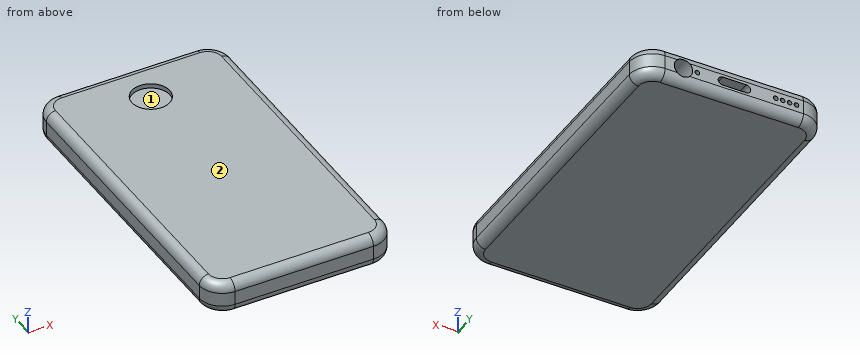
```python
from build123d import *

# Parameters (mm, degrees)
F0_W         = 40
F0_H         = 70
F1_DEPTH     = 7
F2_R         = 5
F3_R         = 2
F4_DEPTH     = 5
F5_T1_DEPTH  = 30
F5_T3_DEPTH  = 60
F5_T6_ANGLE  = 90
F5_T8_ANGLE  = 90
F5_T10_ANGLE = 90
F5_T12_ANGLE = 90
F5_T14_ANGLE = 90
F5_T16_ANGLE = 90
F5_T18_ANGLE = 90
F5_T20_ANGLE = 90
F6_R         = 4.1045895756
F7_DEPTH     = 1
F8_R         = 0.5
F9_DEPTH     = 5
F11_DEPTH    = 5
F12_R        = 0.5
F13_DEPTH    = 5


# Not quite as in the source:
# - a fillet or chamfer that OpenCascade refuses, or shapes differently, is made with other operations: its cross-section is extruded or revolved along the edge and cut away or added


with BuildPart() as f1:
    # F0 (on Top) → F1 (new body)
    with BuildSketch(Plane.XY):
        with Locations((20, 35)):
            Rectangle(F0_W, F0_H)
    extrude(amount=F1_DEPTH)

    # F2
    f2_edges = [f1.edges().sort_by_distance(p)[0] for p in [
        (40, 0, 3.5),
        (0, 0, 3.5),
        (40, 70, 3.5),
        (0, 70, 3.5),
    ]]
    fillet(f2_edges, radius=F2_R)

    # F3 (on face) → F4 (cut)
    with BuildSketch(Plane(origin=(0, 70, 0), x_dir=(-1, 0, 0), z_dir=(0, 1, 0))):
        with Locations((-31, 3.5)):
            Circle(F3_R)
    extrude(amount=-F4_DEPTH, mode=Mode.SUBTRACT)

    # F5: fillet of radius 2 on 16 edges, made by hand

    # F5_s2 → F5_t1 (cut)
    with BuildSketch(Plane.YZ.offset(5)):
        with BuildLine():
            ThreePointArc((68, 7), (69.4142135624, 6.4142135624), (70, 5))
            Line((70, 5), (70, 7))
            Line((70, 7), (68, 7))
        make_face()
        with BuildLine():
            ThreePointArc((68, 0), (69.4142135624, 0.5857864376), (70, 2))
            Line((70, 2), (70, 0))
            Line((70, 0), (68, 0))
        make_face()
        with BuildLine():
            ThreePointArc((2, 0), (0.5857864376, 0.5857864376), (0, 2))
            Line((0, 2), (0, 0))
            Line((0, 0), (2, 0))
        make_face()
        with BuildLine():
            ThreePointArc((2, 7), (0.5857864376, 6.4142135624), (0, 5))
            Line((0, 5), (0, 7))
            Line((0, 7), (2, 7))
        make_face()
    extrude(amount=F5_T1_DEPTH, mode=Mode.SUBTRACT)

    # F5_s4 → F5_t3 (cut)
    with BuildSketch(Plane.XZ.offset(-65)):
        with BuildLine():
            ThreePointArc((0, 2), (0.5857864376, 0.5857864376), (2, 0))
            Line((2, 0), (0, 0))
            Line((0, 0), (0, 2))
        make_face()
        with BuildLine():
            ThreePointArc((0, 5), (0.5857864376, 6.4142135624), (2, 7))
            Line((2, 7), (0, 7))
            Line((0, 7), (0, 5))
        make_face()
        with BuildLine():
            ThreePointArc((38, 0), (39.4142135624, 0.5857864376), (40, 2))
            Line((40, 2), (40, 0))
            Line((40, 0), (38, 0))
        make_face()
        with BuildLine():
            ThreePointArc((38, 7), (39.4142135624, 6.4142135624), (40, 5))
            Line((40, 5), (40, 7))
            Line((40, 7), (38, 7))
        make_face()
    extrude(amount=F5_T3_DEPTH, mode=Mode.SUBTRACT)

    # F5_s5 → F5_t6 (revolve, cut)
    with BuildSketch(Plane.XZ.offset(-65)):
        with BuildLine():
            ThreePointArc((2, 0), (0.5857864376, 0.5857864376), (0, 2))
            Line((0, 2), (0, 0))
            Line((0, 0), (2, 0))
        make_face()
    revolve(axis=Axis((5, 65, 0), (0, 0, -1)), revolution_arc=F5_T6_ANGLE, mode=Mode.SUBTRACT)

    # F5_s7 → F5_t8 (revolve, cut)
    with BuildSketch(Plane.XZ.offset(-5)):
        with BuildLine():
            ThreePointArc((2, 0), (0.5857864376, 0.5857864376), (0, 2))
            Line((0, 2), (0, 0))
            Line((0, 0), (2, 0))
        make_face()
    revolve(axis=Axis((5, 5, 0), (0, 0, 1)), revolution_arc=F5_T8_ANGLE, mode=Mode.SUBTRACT)

    # F5_s9 → F5_t10 (revolve, cut)
    with BuildSketch(Plane.XZ.offset(-65)):
        with BuildLine():
            ThreePointArc((38, 0), (39.4142135624, 0.5857864376), (40, 2))
            Line((40, 2), (40, 0))
            Line((40, 0), (38, 0))
        make_face()
    revolve(axis=Axis((35, 65, 0), (0, 0, 1)), revolution_arc=F5_T10_ANGLE, mode=Mode.SUBTRACT)

    # F5_s11 → F5_t12 (revolve, cut)
    with BuildSketch(Plane.YZ.offset(35)):
        with BuildLine():
            ThreePointArc((2, 0), (0.5857864376, 0.5857864376), (0, 2))
            Line((0, 2), (0, 0))
            Line((0, 0), (2, 0))
        make_face()
    revolve(axis=Axis((35, 5, 0), (0, 0, 1)), revolution_arc=F5_T12_ANGLE, mode=Mode.SUBTRACT)

    # F5_s13 → F5_t14 (revolve, cut)
    with BuildSketch(Plane.XZ.offset(-65)):
        with BuildLine():
            ThreePointArc((0, 5), (0.5857864376, 6.4142135624), (2, 7))
            Line((2, 7), (0, 7))
            Line((0, 7), (0, 5))
        make_face()
    revolve(axis=Axis((5, 65, 7), (0, 0, -1)), revolution_arc=F5_T14_ANGLE, mode=Mode.SUBTRACT)

    # F5_s15 → F5_t16 (revolve, cut)
    with BuildSketch(Plane.XZ.offset(-5)):
        with BuildLine():
            ThreePointArc((0, 5), (0.5857864376, 6.4142135624), (2, 7))
            Line((2, 7), (0, 7))
            Line((0, 7), (0, 5))
        make_face()
    revolve(axis=Axis((5, 5, 7), (0, 0, 1)), revolution_arc=F5_T16_ANGLE, mode=Mode.SUBTRACT)

    # F5_s17 → F5_t18 (revolve, cut)
    with BuildSketch(Plane.XZ.offset(-65)):
        with BuildLine():
            ThreePointArc((38, 7), (39.4142135624, 6.4142135624), (40, 5))
            Line((40, 5), (40, 7))
            Line((40, 7), (38, 7))
        make_face()
    revolve(axis=Axis((35, 65, 7), (0, 0, 1)), revolution_arc=F5_T18_ANGLE, mode=Mode.SUBTRACT)

    # F5_s19 → F5_t20 (revolve, cut)
    with BuildSketch(Plane.YZ.offset(35)):
        with BuildLine():
            ThreePointArc((2, 7), (0.5857864376, 6.4142135624), (0, 5))
            Line((0, 5), (0, 7))
            Line((0, 7), (2, 7))
        make_face()
    revolve(axis=Axis((35, 5, 7), (0, 0, 1)), revolution_arc=F5_T20_ANGLE, mode=Mode.SUBTRACT)

    # F6 (on face) → F7 (cut)
    with BuildSketch(Plane.XY.offset(7)):
        with Locations((20, 60.1752847433)):
            Circle(F6_R)
    extrude(amount=-F7_DEPTH, mode=Mode.SUBTRACT)

    # F8 (on face) → F9 (cut)
    with BuildSketch(Plane(origin=(0, 70, 0), x_dir=(-1, 0, 0), z_dir=(0, 1, 0))):
        with Locations((-28, 3.5)):
            Circle(F8_R)
    extrude(amount=-F9_DEPTH, mode=Mode.SUBTRACT)

    # F10 (on face) → F11 (cut)
    with BuildSketch(Plane(origin=(0, 70, 0), x_dir=(-1, 0, 0), z_dir=(0, 1, 0))):
        with BuildLine():
            Line((-17.383011058, 4.4047813863), (-22.5439444184, 4.4047813863))
            ThreePointArc((-22.5439444184, 4.4047813863), (-23.4822960338, 3.4664297709), (-22.5439444184, 2.5280781556))
            Line((-22.5439444184, 2.5280781556), (-17.383011058, 2.5280781556))
            ThreePointArc((-17.383011058, 2.5280781556), (-16.4446594426, 3.4664297709), (-17.383011058, 4.4047813863))
        make_face()
    extrude(amount=-F11_DEPTH, mode=Mode.SUBTRACT)

    # F12 (on face) → F13 (cut)
    with BuildSketch(Plane(origin=(0, 70, 0), x_dir=(-1, 0, 0), z_dir=(0, 1, 0))):
        with Locations((-6.5, 3.5)):
            Circle(F12_R)
        with Locations((-8, 3.5)):
            Circle(F12_R)
        with Locations((-9.5, 3.5)):
            Circle(F12_R)
        with Locations((-11, 3.5)):
            Circle(F12_R)
    extrude(amount=-F13_DEPTH, mode=Mode.SUBTRACT)


solid = f1.part
```
Geometry: final body of the model. Coordinates: model frame, mm. Face numbers are marked on the shaded views. Give positions to 0.01 mm unless a question says otherwise; leave off trailing zeros. Loops run counter-clockwise (first coordinate to the right, second up) from the corner with the lowest first, then second, coordinate; pieces in that order, holes last. Notation, with made-up numbers: (-30, 43) -> (-21, 43) arc R15 ccw to (-21, 48) -> close; hole circle Ø5 at (-2, -14.75). An arc over 180 degrees is marked (long way). Use CSV: the item, a comma, the result in double quotes.
(1) Cut plane A-A (x = 20). Output: boundary loops of the cut face in (y, z).
From the geometry:
outline,"(0, 2) arc R2 ccw to (2, 0) -> (68, 0) arc R2 ccw to (70, 2) -> (70, 2.53) -> (65, 2.53) -> (65, 4.4) -> (70, 4.4) -> (70, 5) arc R2 ccw to (68, 7) -> (64.28, 7) -> (64.28, 6) -> (56.07, 6) -> (56.07, 7) -> (2, 7) arc R2 ccw to (0, 5) -> close"
(2) Pull-direction query (Y, two-part tool) for the marked faces 1 and 2; classes: released by +Y, released by -Y, zero draft, split by the parting line, or undercut.
From the geometry:
face 1,"undercut"
face 2,"zero draft"
(3) First-contact query: P1, Ø0.6, axis at x = 18.5, z = 3, coming from the +Y side; P2, Ø2.5, axis at x = 20, y = 60, coming from the +Z side. Flat tips, straight axial feed; report the tip coordinate or a pass-through.
From the geometry:
P1,"y = 65"
P2,"z = 6"
(4) Cut plane B-B (x = 31). Output: boundary loops of the cut face in (y, z), plus the area to 3 significant figures.
From the geometry:
outline,"(0, 2) arc R2 ccw to (2, 0) -> (68, 0) arc R2 ccw to (69.94, 1.5) -> (65, 1.5) -> (65, 5.5) -> (69.94, 5.5) arc R2 ccw to (68, 7) -> (2, 7) arc R2 ccw to (0, 5) -> close"
area,"467 mm^2"
(5) Ray query, line 1 along Z through (x, y) = (31, 66); line 2 along Z through (x, y) = (8, 68); line 3 along Y through (x, z) = (21, 3). Return the intervals inside material, ascending. Write a range as [from, to].
From the geometry:
line 1,"[0, 1.5], [5.5, 7]"
line 2,"[0, 3], [4, 7]"
line 3,"[0, 65]"
